The model under review builds one solid part; all positions refer to its coordinate system, in mm. A direction names the side the tool comes from. Round coordinates to 2 decimals unless told otherwise and drop trailing zeros. Order: outer loops, then holes, each group sorted by start corner. A loop starts at its lowest first (then second) coordinate and runs counter-clockwise, first axis right, second up. Notation, with made-up numbers: (-17.5, -18) - (16.5, -18) arc R21 ccw to (16.5, 6) - close; hole circle Ø5 at (71, 64.5). An arc over 180 degrees is marked (long way). One line per question, with ' | ' between items. Start each with the question number.
Item 1: Insertion check: pin 1 Ø11.5 at (y, z) = (24, -0.5) entering from +X; pin 2 Ø1.5 at (x, z) = (21.5, 7.5) entering from +Y; pin 3 Ø11.5 at (x, z) = (12.7, 12.7) entering from +Y; pin 4 Ø10 at (x, z) = (19, 10) entering from -Y. Each pin has a flat end and moves straight along its axis. Give the tip position at first contact, or say it passes through.
Item 2: Draft analysis for pull direction Y (two halves, no side actions). For faces 1 (the face through (2.354, 12.543, -16.265)), 2 (the face through (27, 4.775, 0)), 3 (the face through (35.69, 2.35, -10.07)), 4 (the face through (2.35, 35.69, 10.07)), state which applies: +Y half, -Y half, draft (parallel to the pull), parting line (faces both ways), or undercut.
Item 3: For L1, parallel to Z at x = 3.2, y = 12.7; L2, parallel to X at y = 1.1, z = 12.7; L3, parallel to X at y = 3, z = 12, list the stretches that pass through material, from the lowest coordinate up. Write a range as [from, to].
Item 4: Add section A-A on x = 38.1. State the section outline as (y, z) points, and give its area (3 significant figures).
Item 5: Tool access review of faces 5 (the face through (2.354, 12.543, 9.135)), 6 (the face through (4.775, 27, 0)): name each direction out of +Z, -Z, +X, -X, +Y, -Y from which nothing blocks a thin tool from reaching the whole face with its end or side.
Item 6: Add section D-D on z = 19. State the section outline as (x, y) points (3 decimals), and give its area (3 significant figures).
Item 7: Add section B-B on z = 12.7. State the section outline as (x, y) points (3 decimals).
from build123d import *

# Parameters (mm, degrees)
BOSS_EXTRUDE1_DEPTH = 23.8125
SKETCH2_R           = 3.5687
CUT_EXTRUDE1_DEPTH  = 76.685633751
SKETCH3_R           = 3.5687
CUT_EXTRUDE2_DEPTH  = 76.685633751


with BuildPart() as part:
    # Sketch1 → Boss-Extrude1 (new, symmetric)
    with BuildSketch(Plane.XY):
        with BuildLine():
            Line((0, 0), (0, 50.8))
            ThreePointArc((0, 50.8), (3.376576302, 49.401376302), (4.7752, 46.0248))
            Line((4.7752, 46.0248), (4.7752, 7.9502))
            ThreePointArc((4.7752, 7.9502), (5.70513597, 5.70513597), (7.9502, 4.7752))
            Line((7.9502, 4.7752), (46.0248, 4.7752))
            ThreePointArc((46.0248, 4.7752), (49.401376302, 3.376576302), (50.8, 0))
            Line((50.8, 0), (0, 0))
        make_face()
    extrude(amount=BOSS_EXTRUDE1_DEPTH, both=True)

    # Sketch2 → Cut-Extrude1 (cut, through all)
    with BuildSketch(Plane(origin=(0, 0, 0), x_dir=(1, 0, 0), z_dir=(0, 1, 0))):
        with Locations(Location((12.7, -12.7, 0), (0, 0, 90))):
            Circle(SKETCH2_R)
        with Locations(Location((38.1, -12.7, 0), (0, 0, 90))):
            Circle(SKETCH2_R)
        with Locations(Location((12.7, 12.7, 0), (0, 0, 90))):
            Circle(SKETCH2_R)
        with Locations(Location((38.1, 12.7, 0), (0, 0, 90))):
            Circle(SKETCH2_R)
    extrude(amount=CUT_EXTRUDE1_DEPTH, mode=Mode.SUBTRACT)

    # Sketch3 → Cut-Extrude2 (cut, through all)
    with BuildSketch(Plane(origin=(0, 0, 0), x_dir=(0, 0, -1), z_dir=(1, 0, 0))):
        with Locations(Location((-12.7, 12.7, 0), (0, 0, 180))):
            Circle(SKETCH3_R)
        with Locations(Location((-12.7, 38.1, 0), (0, 0, 180))):
            Circle(SKETCH3_R)
        with Locations(Location((12.7, 12.7, 0), (0, 0, 180))):
            Circle(SKETCH3_R)
        with Locations(Location((12.7, 38.1, 0), (0, 0, 180))):
            Circle(SKETCH3_R)
    extrude(amount=CUT_EXTRUDE2_DEPTH, mode=Mode.SUBTRACT)


solid = part.part
Determined:
1) pin 1: x = 4.78 | pin 2: y = 4.78 | pin 3: y = 4.94 | pin 4: y = 0
2) face 1: undercut | face 2: +Y half | face 3: draft | face 4: undercut
3) L1: [-23.81, -16.27], [-9.13, 9.13], [16.27, 23.81] | L2: [0, 9.13], [16.27, 34.53], [41.67, 50.67] | L3: [0, 9.2], [16.2, 34.6], [41.6, 49.74]
4) outline: (0, -23.81) - (4.78, -23.81) - (4.78, -16.27) - (0, -16.27) - close; (0, -9.13) - (4.78, -9.13) - (4.78, 9.13) - (0, 9.13) - close; (0, 16.27) - (4.78, 16.27) - (4.78, 23.81) - (0, 23.81) - close | area: 159 mm2
5) face 5: +X, -X | face 6: +Z, -Z, +X, +Y
6) outline: (0, 0) - (50.8, 0) arc R4.775 ccw to (46.025, 4.775) - (7.95, 4.775) arc R3.175 cw to (4.775, 7.95) - (4.775, 46.025) arc R4.775 ccw to (0, 50.8) - close | area: 455 mm2
7) outline: (0, 0) - (9.131, 0) - (9.131, 4.775) - (7.95, 4.775) arc R3.175 cw to (4.775, 7.95) - (4.775, 9.131) - (0, 9.131) - close; (0, 16.269) - (4.775, 16.269) - (4.775, 34.531) - (0, 34.531) - close; (0, 41.669) - (4.775, 41.669) - (4.775, 46.025) arc R4.775 ccw to (0, 50.8) - close; (16.269, 0) - (34.531, 0) - (34.531, 4.775) - (16.269, 4.775) - close; (41.669, 0) - (50.8, 0) arc R4.775 ccw to (46.025, 4.775) - (41.669, 4.775) - close
